```python
from build123d import *

# Parameters (mm, degrees)
EXTRUDE_1_DEPTH     = 1
CHAMFER_2_SIZE      = 3
CHAMFER_1_SIZE      = 0.6
SKETCH_2_W          = 16
SKETCH_2_H          = 26
CUT_EXTRUDE_1_DEPTH = 10
CHAMFER_3_SIZE      = 3
CHAMFER_4_SIZE      = 0.8
SKETCH_3_W          = 6
SKETCH_3_H          = 6
EXTRUDE_2_DEPTH     = 3
SKETCH_4_R          = 1.2
CUT_EXTRUDE_2_DEPTH = 5
SKETCH_5_R          = 2.05
CUT_EXTRUDE_3_DEPTH = 2
FILLET_1_R          = 2
SKETCH_7_W          = 3.1
SKETCH_7_H          = 5.1
CUT_EXTRUDE_4_DEPTH = 2
FILLET_2_R          = 0.4
CHAMFER_5_SIZE      = 0.8


with BuildPart() as part:
    # 草图1 → 凸台-拉伸1 (new body)
    with BuildSketch(Plane(origin=(0, 0, 0), x_dir=(1, 0, 0), z_dir=(0, 1, 0))):
        Polygon((0, 0), (50, 0), (50, 30), (30, 50), (0, 20), align=None)
    extrude(amount=EXTRUDE_1_DEPTH)

    # 倒角2
    chamfer_2_edges = [part.edges().sort_by_distance(p)[0] for p in [
        (50, 0.5, 0),
    ]]
    chamfer(chamfer_2_edges, length=CHAMFER_2_SIZE)

    # 倒角1
    chamfer_1_edges = [part.edges().sort_by_distance(p)[0] for p in [
        (40, 1, -40),
        (50, 1, -16.5),
        (48.5, 1, -1.5),
        (15, 1, -35),
        (0, 1, -10),
        (23.5, 1, 0),
    ]]
    chamfer(chamfer_1_edges, length=CHAMFER_1_SIZE)

    # 草图2 → 切除-拉伸1 (cut)
    with BuildSketch(Plane(origin=(0, 1, 0), x_dir=(1, 0, 0), z_dir=(0, 1, 0))):
        with Locations((30, 25)):
            Rectangle(SKETCH_2_W, SKETCH_2_H)
    extrude(amount=-CUT_EXTRUDE_1_DEPTH, mode=Mode.SUBTRACT)

    # 倒角3
    chamfer_3_edges = [part.edges().sort_by_distance(p)[0] for p in [
        (22, 0.5, -12),
        (38, 0.5, -38),
    ]]
    chamfer(chamfer_3_edges, length=CHAMFER_3_SIZE)

    # 倒角4
    chamfer_4_edges = [part.edges().sort_by_distance(p)[0] for p in [
        (22, 1, -26.5),
        (38, 1, -23.5),
        (28.5, 1, -38),
        (31.5, 1, -12),
        (36.5, 1, -36.5),
        (23.5, 1, -13.5),
    ]]
    chamfer(chamfer_4_edges, length=CHAMFER_4_SIZE)

    # 草图3 → 凸台-拉伸2 (add)
    with BuildSketch(Plane.XZ):
        with Locations((8, -3)):
            Rectangle(SKETCH_3_W, SKETCH_3_H)
        with Locations((47, -21)):
            Rectangle(SKETCH_3_W, SKETCH_3_H)
    extrude(amount=EXTRUDE_2_DEPTH)

    # 草图4 → 切除-拉伸2 (cut, through all)
    with BuildSketch(Plane.XZ.offset(3)):
        with Locations((8, -3.05)):
            Circle(SKETCH_4_R)
        with Locations((47, -21)):
            Circle(SKETCH_4_R)
    extrude(amount=-CUT_EXTRUDE_2_DEPTH, mode=Mode.SUBTRACT)

    # 草图5 → 切除-拉伸3 (cut)
    with BuildSketch(Plane(origin=(0, 1, 0), x_dir=(1, 0, 0), z_dir=(0, 1, 0))):
        with Locations((8, 3.05)):
            Circle(SKETCH_5_R)
        with Locations((47, 21)):
            Circle(SKETCH_5_R)
    extrude(amount=-CUT_EXTRUDE_3_DEPTH, mode=Mode.SUBTRACT)

    # 圆角1
    fillet_1_edges = [part.edges().sort_by_distance(p)[0] for p in [
        (5, -1.5, -6),
        (11, -1.5, -6),
        (44, -1.5, -18),
        (44, -1.5, -24),
    ]]
    fillet(fillet_1_edges, radius=FILLET_1_R)

    # 草图7 → 切除-拉伸4 (cut)
    with BuildSketch(Plane(origin=(0, 1, 0), x_dir=(1, 0, 0), z_dir=(0, 1, 0))):
        with Locations((37.947463912, 5.75)):
            Rectangle(SKETCH_7_W, SKETCH_7_H)
        with Locations((22.050353573, 5.75)):
            Rectangle(SKETCH_7_W, SKETCH_7_H)
    extrude(amount=-CUT_EXTRUDE_4_DEPTH, mode=Mode.SUBTRACT)

    # 圆角2
    fillet_2_edges = [part.edges().sort_by_distance(p)[0] for p in [
        (20.500353573, 0.5, -8.3),
        (23.600353573, 0.5, -8.3),
        (23.600353573, 0.5, -3.2),
        (20.500353573, 0.5, -3.2),
        (39.497463912, 0.5, -3.2),
        (36.397463912, 0.5, -3.2),
        (36.397463912, 0.5, -8.3),
        (39.497463912, 0.5, -8.3),
    ]]
    fillet(fillet_2_edges, radius=FILLET_2_R)

    # 倒角5
    chamfer_5_edges = [part.edges().sort_by_distance(p)[0] for p in [
        (37.947463912, 1, -3.2),
        (36.397463912, 1, -5.75),
        (37.947463912, 1, -8.3),
        (39.497463912, 1, -5.75),
        (23.600353573, 1, -5.75),
        (22.050353573, 1, -3.2),
        (22.050353573, 1, -8.3),
        (20.500353573, 1, -5.75),
        (36.514621199, 1, -3.317157288),
        (36.514621199, 1, -8.182842712),
        (39.380306624, 1, -8.182842712),
        (39.380306624, 1, -3.317157288),
        (23.483196285, 1, -3.317157288),
        (23.483196285, 1, -8.182842712),
        (20.61751086, 1, -8.182842712),
        (20.61751086, 1, -3.317157288),
    ]]
    chamfer(chamfer_5_edges, length=CHAMFER_5_SIZE)


solid = part.part
```
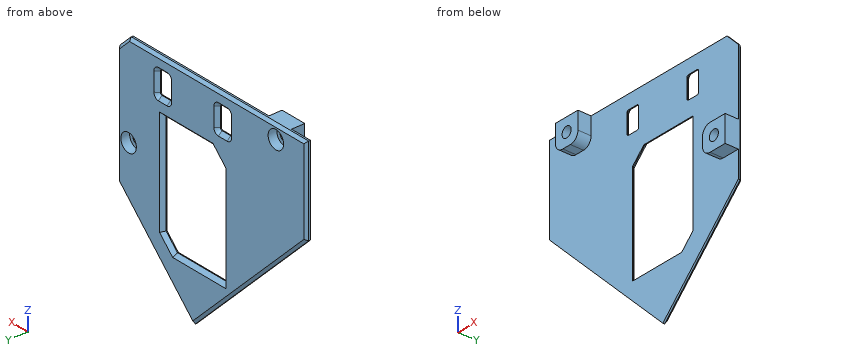
Geometry: final body of the model. Coordinates: model frame, mm. Give positions to 0.01 mm unless a question says otherwise; leave off trailing zeros. Loops run counter-clockwise (first coordinate to the right, second up) from the corner with the lowest first, then second, coordinate; pieces in that order, holes last. Notation, with made-up numbers: (59, 68.5) -> (82, 68.5) arc R27 cw to (82, 107.5) -> close; hole circle Ø7 at (37, 55). An arc over 180 degrees is marked (long way). Use one line per item in the form item = value.
Item 1: Line query: probe 1 along X at (y, z) = (0.25, -21); probe 2 along X at (y, z) = (0.55, -21); probe 3 along X at (y, z) = (0.05, -3.05). Output: solid intervals per line, ascending.
A:
probe_1 = 1 to 21.95, 38.05 to 44.95, 49.05 to 50
probe_2 = 1.21 to 21.65, 38.35 to 44.95, 49.05 to 49.85
probe_3 = 0 to 5.95, 10.05 to 50
Item 2: Section query D-D on z = -21. Output: boundary loops of the cut face in (x, y), and give its area (3 significant figures).
A:
outline = (1, 0) -> (22, 0) -> (22, 0.2) -> (21.2, 1) -> (1.85, 1) -> (1, 0.4) -> close; (38, 0) -> (44, 0) -> (44, -3) -> (45.8, -3) -> (45.8, -1) -> (44.95, -1) -> (44.95, 1) -> (38.8, 1) -> (38, 0.2) -> close; (48.2, -3) -> (50, -3) -> (50, 0.4) -> (49.4, 1) -> (49.05, 1) -> (49.05, -1) -> (48.2, -1) -> close
area = 36.9 mm^2
Item 3: Pin query (flat end, axial travel): P1, Ø1.5, axis at x = 48.5, y = -1, coming from the -Z side; P2, Ø1.5, axis at y = -2, z = -2.5, coming from the -X side; P3, Ø3, axis at x = 22.5, z = -39, coming from the -Y side. Return the tip coordinate at first contact, or that it passes through.
A:
P1 = -24
P2 = 5
P3 = 0
Item 4: Section query A-A on z = -7. Output: boundary loops of the cut face in (x, y), and give its area (3 significant figures).
A:
outline = (0, 0) -> (20.5, 0) -> (20.5, 0.2) -> (19.7, 1) -> (0.6, 1) -> (0, 0.4) -> close; (23.6, 0) -> (36.4, 0) -> (36.4, 0.2) -> (35.6, 1) -> (24.4, 1) -> (23.6, 0.2) -> close; (39.5, 0) -> (50, 0) -> (50, 0.4) -> (49.4, 1) -> (40.3, 1) -> (39.5, 0.2) -> close
area = 42.2 mm^2
Item 5: Section query C-C on x = 42. Output: boundary loops of the cut face in (y, z).
A:
outline = (0, -38) -> (0.4, -38) -> (1, -37.15) -> (1, -0.6) -> (0.4, 0) -> (0, 0) -> close
Item 6: Section query B-B on z = -28.5. Output: boundary loops of the cut face in (x, y), and give its area (3 significant figures).
A:
outline = (8.5, 0) -> (22, 0) -> (22, 0.2) -> (21.2, 1) -> (9.35, 1) -> (8.5, 0.4) -> close; (38, 0) -> (50, 0) -> (50, 0.4) -> (49.4, 1) -> (38.8, 1) -> (38, 0.2) -> close
area = 24.4 mm^2
